Could you check a few things on this model? Use its own coordinates, in mm. Face numbers are marked on the shaded views. A direction names the side the tool comes from. Coordinates: 2 decimals unless noted, no trailing zeros. Order: outer loops, then holes, each group sorted by start corner. A loop starts at its lowest first (then second) coordinate and runs counter-clockwise, first axis right, second up. Notation, with made-up numbers: (51, 67.25) -> (73, 67.25) arc R28 ccw to (73, 87.25) -> close; hole circle Ø1 at (69, -27). An arc over 180 degrees is marked (long way). Use a Markdown table: item, result. Add a question column.
1) If I drill on L1, parallel to Z at x = 20, y = 5; L2, parallel to X at y = -21.5, z = 58; L3, parallel to X at y = -32, z = 17.5, over which ranges is the centre line in solid material (lowest first)? Write a range as [from, to].
2) Will these pins go through, and if not, where does the flat tip stop? pin 1 Ø8 at (x, z) = (11.5, 89) entering from -Y; pin 2 Ø12 at (x, z) = (-35.5, 28.5) entering from -Y; pin 3 Ø12 at (x, z) = (-28.5, 107) entering from -Y.
3) Thinking about a two-plate mould opening in Z: for the marked faces 4, 5 and 6, which applies, +Z half, -Z half, draft (parallel to the pull), parting line (faces both ways), or undercut?
4) If we section it at B-B (x = -153.5): Write out the boundary of the cut face in (y, z), plus the area to 3 significant figures.
5) Which directions (+Z, -Z, +X, -X, +Y, -Y) give clear straight access to the entire face, cutting with the end or side of a thin tool? Please do the marked faces 1, 2 and 3.
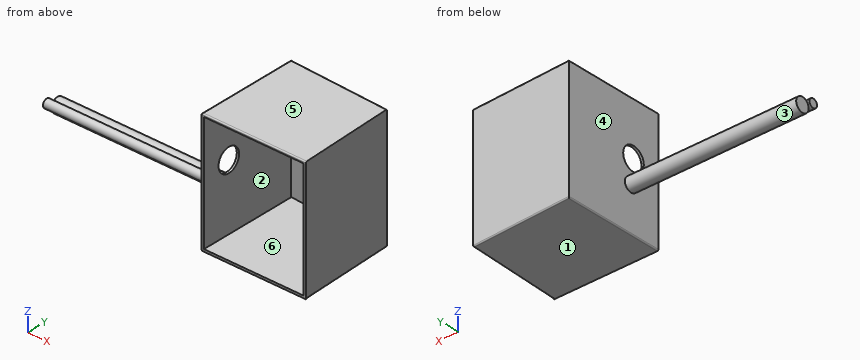
```python
from build123d import *

# Parameters (mm, degrees)
F1_DEPTH  = 132.334
F2_T      = -2.54
F3_DEPTH  = 0.762
F5_D      = 25.4
F5_DEPTH  = 5.08
F5_TIP    = 7.6309298617
F9_R      = 1.2264204897
F7_R      = 7.7162508116
F7_R_2    = 4.6438728955
F10_DEPTH = 189.738


with BuildPart() as f1:
    # F0 (on Top) → F1 (new body)
    with BuildSketch(Plane.XY):
        Polygon((52.318636328, 57.9638108611), (-57.1821704507, 63.2404088974), (-57.1821704507, -47.161385417), (56.8056404591, -47.161385417), align=None)
    extrude(amount=F1_DEPTH)

    # F2
    f2_openings = [f1.faces().sort_by_distance(p)[0] for p in [
        (-0.188265, -47.161385, 66.167),
    ]]
    offset(amount=F2_T, openings=f2_openings)

    # F3 (add): a face of the model
    f3_faces = [f1.faces().sort_by_distance(p)[0] for p in [
        (-55.4355878276, -47.161385417, 66.167),
    ]]
    extrude(f3_faces, amount=-F3_DEPTH)

    # F5 (one way)
    with BuildSketch(Plane.YZ.offset(-54.6421704507)):
        with Locations((-16.4339449257, 74.0607306361)):
            Circle(F5_D / 2)
    extrude(amount=-F5_DEPTH, mode=Mode.SUBTRACT)
    with Locations(Plane.YZ.offset(-54.6421704507)):
        with Locations((-16.4339449257, 74.0607306361)):
            with Locations((0, 0, -(F5_DEPTH + F5_TIP / 2))):  # 118° drill point
                Cone(0, F5_D / 2, F5_TIP, mode=Mode.SUBTRACT)

    # F9
    f9_edges = [f1.edges().sort_by_distance(p)[0] for p in [
        (-57.18217, 8.039512, 132.334),
        (-2.431767, 60.60211, 132.334),
        (-0.188265, -47.161385, 132.334),
        (-57.18217, 8.039512, 0),
        (54.545876, 5.782213, 0),
        (-2.431767, 60.60211, 0),
    ]]
    fillet(f9_edges, radius=F9_R)

    # F7 (on face) → F10 (join)
    with BuildSketch(Plane.YZ.offset(-54.6421704507)):
        with Locations((-13.5401813313, 47.8832386434)):
            Circle(F7_R)
        with Locations((-26.8557239324, 55.4966442287)):
            Circle(F7_R_2)
    extrude(amount=-F10_DEPTH)


solid = f1.part
```
Answer sheet:
| question | item | result |
|---|---|---|
| 1 | L1 | [0, 2.54], [129.79, 132.33] |
| 1 | L2 | [-57.18, -54.64], [53.17, 55.71] |
| 1 | L3 | [-57.18, -54.64], [53.62, 56.16] |
| 2 | pin 1 | y = 57.2 |
| 2 | pin 2 | y = 59.36 |
| 2 | pin 3 | y = 59.03 |
| 3 | face 4 | draft |
| 3 | face 5 | +Z half |
| 3 | face 6 | undercut |
| 4 | outline | circle Ø9.29 at (-26.86, 55.5); circle Ø15.43 at (-13.54, 47.88) |
| 4 | area | 255 mm2 |
| 5 | face 1 | -Z, +X, -X, +Y, -Y |
| 5 | face 2 | -Y |
| 5 | face 3 | -X |
